CAD build for the part. Positions are in the model's coordinates, mm. Face numbers are marked on the shaded views. A direction names the side the tool comes from. Coordinates: 2 decimals unless noted, no trailing zeros. Write each loop counter-clockwise with the first axis right and the second up, starting at its lowest first coordinate (ties: lowest second). Pieces come first, ordered by that corner, then holes. Notation, with made-up numbers: (66, 30.5) - (99, 30.5) arc R33 ccw to (99, 62.5) - close; hole circle Ø11 at (-18.5, 60). An arc over 180 degrees is marked (long way). Answer in a Markdown table with one row per item. Add a question column.
Q1. Band-saw the part on D-D (x = -3.5). List the corners of the cut face in (y, z).
Q2. 3-axis set-ups, long thin cutter, end or side, ignore diameter. For the marked faces 1, 2 and 3: which of +Z, -Z, +X, -X, +Y, -Y reach the whole face in a straight line?
Q3. Two-plate mould, pull along X, no slides. Class the marked faces 4, 5 and 6: +X half, -X half, draft (parallel to the pull), parting line (faces both ways), or undercut.
Q4. Drill centre lines: line 1 along X through (y, z) = (17, -10.5); line 2 along X through (y, z) = (42.1, -2.25); line 3 along Y through (x, z) = (-10.1, -2). Where is each one in solid material? Low to high. Write a range as from..to.
Q5. Band-saw the part on B-B (y = 42.1). List the corners of the cut face in (x, z), and give its area (3 significant figures).
Q6. Band-saw the part on C-C (z = -4). List the corners of the cut face in (x, y), and give its area (3 significant figures).
Q7. Pin check, flat tips, straight feed: pin 1 (3.5 mm diameter, centred on x = -13, z = -7.5, fed in from -Y); pin 2 (3 mm diameter, centred on x = -5.5, y = 43.5, fed in from -Z); pin 3 (1.5 mm diameter, centred on y = 13, z = -5.5, fed in from +X). Stop position of each tip, or through.
Q8. Band-saw the part on A-A (x = -10.1). List the corners of the cut face in (y, z).
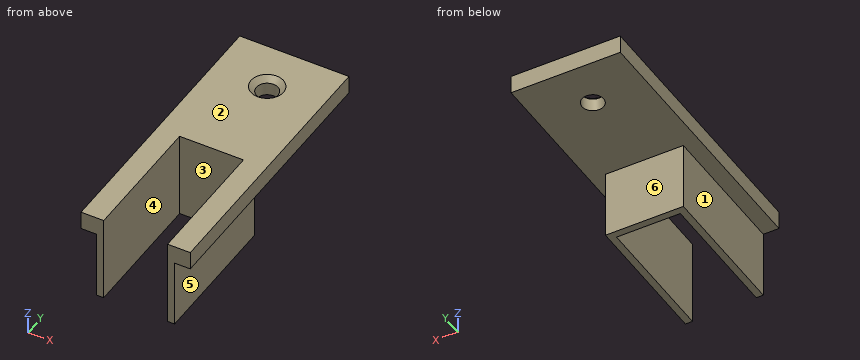
Autodesk Inventor part; units mm, degrees
ref_plane "YZ Plane" through (0, 0, 0) normal (1, 0, 0) x (0, 1, 0)
ref_plane "XZ Plane" through (0, 0, 0) normal (0, 1, 0) x (-1, 0, 0)
ref_plane "XY Plane" through (0, 0, 0) normal (0, 0, 1) x (1, 0, 0)
sketch "Boceto1" plane through (0, 0, 0) normal (0, 0, 1) x (1, 0, 0)
  line L0 (0, 50.8) -> (-20.2, 50.8)
  line L1 (-20.2, 50.8) -> (-20.2, 0)
  line L2 (-20.2, 0) -> (0, 0)
  line L3 (0, 0) -> (0, 50.8)
  dimension "d0" = 50.8
  dimension "d1" = 20.2
extrude "Extrusión1" add sketch "Boceto1" against normal blind 3.4
sketch "Boceto3" plane through (0, 0, 0) normal (0, 0, -1) x (-1, 0, 0)
  line L0 (20.2, 50.8) -> (0, 50.8) construction
  line L1 (0, 50.8) -> (0, 0) construction
  circle A0 centre (10.1, 42.1) radius 2
  line L2 (20.2, 0) -> (20.2, 50.8)
  dimension "d20" = 4
  dimension "d21" = 10.1
  dimension "d23" = 8.7
hole "Agujero3" at (-10.1, 42.1, 0) direction (0, 0, -1) diameter 4 end through all countersink diameter 6 countersink angle 90
sketch "Boceto6" plane through (0, 0, -3.4) normal (0, 0, -1) x (-1, 0, 0)
  line L0 (0, 0) -> (20.2, 0)
  line L1 (2.9, 0) -> (2.9, 25.6)
  line L2 (2.9, 25.6) -> (17.3, 25.6)
  line L3 (17.3, 25.6) -> (17.3, 0)
  line L4 (16, 0) -> (16, 24.3)
  line L5 (16, 24.3) -> (4.2, 24.3)
  line L6 (4.2, 24.3) -> (4.2, 0)
  line L7 (0, 50.8) -> (0, 0)
  line L8 (20.2, 0) -> (20.2, 50.8)
  circle A0 centre (10.1, 42.1) radius 2
  point P0 (4.2, 0)
  point P1 (16, 0)
  dimension "d40" = 1.3
  dimension "d50" = 14.4
  dimension "d51" = 2.9
  dimension "d52" = 2.9
  dimension "d54" = 25.6
  dimension "d55" = 16.5
extrude "Extrusión3" add sketch "Boceto6" along normal blind 12.7 contours L1 L2 L3 L0 L4 L5 L6
sketch "Boceto7" plane through (0, 0, -3.4) normal (0, 0, -1) x (-1, 0, 0)
  line L0 (16, 24.3) -> (16, 0)
  line L1 (4.2, 24.3) -> (16, 24.3)
  line L2 (16, 24.3) -> (16, 0)
  line L3 (16, 0) -> (4.2, 0)
  line L4 (4.2, 0) -> (4.2, 24.3)
  point P0 (0, 0)
extrude "Extrusión4" cut sketch "Boceto7" against normal blind 10
properties part number "PLU-45 TAPÓN ENCUENTRO CORREDERA (2)" material "Plástico ABS"
Checked values:
| question | item | result |
|---|---|---|
| 1 | outline | (0, -16.1) - (25.6, -16.1) - (25.6, -3.4) - (50.8, -3.4) - (50.8, 0) - (0, 0) - close |
| 2 | face 1 | -Z, -X, +Y, -Y |
| 2 | face 2 | +Z, +X, -X, +Y, -Y |
| 2 | face 3 | +Z, -Z, -Y |
| 3 | face 4 | undercut |
| 3 | face 5 | +X half |
| 3 | face 6 | draft |
| 4 | line 1 | x = -17.3..-16, -4.2..-2.9 |
| 4 | line 2 | x = -20.2..-12.1, -8.1..0 |
| 4 | line 3 | y = 24.3..40.1, 44.1..50.8 |
| 5 | outline | (-20.2, -3.4) - (-12.1, -3.4) - (-12.1, -1) - (-13.1, 0) - (-20.2, 0) - close; (-8.1, -3.4) - (0, -3.4) - (0, 0) - (-7.1, 0) - (-8.1, -1) - close |
| 5 | area | 54.1 mm² |
| 6 | outline | (-17.3, 0) - (-16, 0) - (-16, 24.3) - (-4.2, 24.3) - (-4.2, 0) - (-2.9, 0) - (-2.9, 25.6) - (-17.3, 25.6) - close |
| 6 | area | 81.9 mm² |
| 7 | pin 1 | stops at y = 24.3 |
| 7 | pin 2 | stops at z = -3.4 |
| 7 | pin 3 | stops at x = -2.9 |
| 8 | outline | (24.3, -16.1) - (25.6, -16.1) - (25.6, -3.4) - (40.1, -3.4) - (40.1, -1) - (39.1, 0) - (24.3, 0) - close; (44.1, -3.4) - (50.8, -3.4) - (50.8, 0) - (45.1, 0) - (44.1, -1) - close |
